Check sheet for the modelled part. Datum: model origin and axes. Units: mm. Face numbers are marked on the shaded views. A direction names the side the tool comes from. Coordinates: 2 decimals unless noted, no trailing zeros. Write each loop counter-clockwise with the first axis right and the second up, starting at its lowest first coordinate (ties: lowest second). Pieces come first, ordered by that corner, then holes. Notation, with made-up numbers: (74, 67) - (96, 67) arc R10 cw to (96, 71) - close; hole circle Ø6 at (-39, 87.25). An arc over 180 degrees is marked (long way). Use one line per item in the form item = value. Start each with the question number.
1. Cross-section at B-B on y = 7. Record the boundary of the cut face in (x, z).
2. Cross-section at C-C on z = -28.8. Record the boundary of the cut face in (x, y).
3. Cross-section at D-D on x = 4.5. Record the boundary of the cut face in (y, z).
4. Tool access check on the marked faces 1, 2 and 3. Record the directions out of +Z, -Z, +X, -X, +Y, -Y that give a thin tool (end or side, any length) a straight path to the whole face; none if there is none.
5. Go/stop test with flat-tipped pins: pin 1 Ø3 at (x, z) = (11, 43) entering from -Y; pin 2 Ø8 at (y, z) = (6, -21.5) entering from -X; pin 3 Ø1.5 at (x, y) = (7.5, 13.5) entering from -Z. Record where each tip stops, or that it passes through.
6. Scan lines: line 1 along Z through (x, y) = (-6.5, 11); line 2 along Z through (x, y) = (15, 6); line 3 along Y through (x, z) = (0.5, 49). Record each from-to range of solid material in increasing order.
7. Cross-section at A-A on x = 0. Record the boundary of the cut face in (y, z), then the cut area to 3 significant figures.
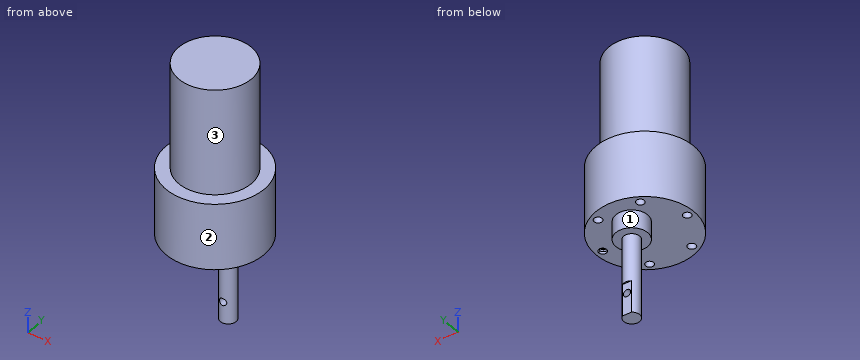
```python
from build123d import *

# Parameters (mm, degrees)
SKETCH1_R           = 18.5
BOSS_EXTRUDE1_DEPTH = 25
SKETCH2_R           = 6
BOSS_EXTRUDE2_DEPTH = 6.8
SKETCH3_R           = 3
BOSS_EXTRUDE3_DEPTH = 30
CUT_EXTRUDE1_DEPTH  = 12
SKETCH5_R           = 13.7
BOSS_EXTRUDE4_DEPTH = 40
SKETCH6_R           = 1.5
CUT_EXTRUDE2_DEPTH  = 3.2
THREAD1_PITCH       = 1.058333333
SKETCH7_R           = 1.350457069
CUT_EXTRUDE3_DEPTH  = 10


with BuildPart() as part:
    # Sketch1 → Boss-Extrude1 (new body)
    with BuildSketch(Plane.XY):
        Circle(SKETCH1_R)
    extrude(amount=BOSS_EXTRUDE1_DEPTH)

    # Sketch2 → Boss-Extrude2 (add)
    with BuildSketch(Plane(origin=(0, 0, 0), x_dir=(-1, 0, 0), z_dir=(0, 0, -1))):
        with Locations(Location((0, 7, 0), (0, 0, 180))):
            Circle(SKETCH2_R)
    extrude(amount=BOSS_EXTRUDE2_DEPTH)

    # Sketch3 → Boss-Extrude3 (add)
    with BuildSketch(Plane(origin=(0, 0, -6.8), x_dir=(-1, 0, 0), z_dir=(0, 0, -1))):
        with Locations((0, 7)):
            Circle(SKETCH3_R)
    extrude(amount=BOSS_EXTRUDE3_DEPTH)

    # Sketch4 → Cut-Extrude1 (cut)
    with BuildSketch(Plane(origin=(0, 0, -36.8), x_dir=(-1, 0, 0), z_dir=(0, 0, -1))):
        Polygon((-80.661429966, 9.5), (-1.658312395, 9.5), (1.658312395, 9.5), (80.661429966, 9.5), (80.661429966, 167.506235142), (-80.661429966, 167.506235142), align=None)
    extrude(amount=-CUT_EXTRUDE1_DEPTH, mode=Mode.SUBTRACT)

    # Sketch5 → Boss-Extrude4 (add)
    with BuildSketch(Plane.XY.offset(25)):
        Circle(SKETCH5_R)
    extrude(amount=BOSS_EXTRUDE4_DEPTH)

    # Sketch6 → Cut-Extrude2 (cut)
    with BuildSketch(Plane(origin=(0, 0, 0), x_dir=(-1, 0, 0), z_dir=(0, 0, -1))):
        with Locations((-15.75, 0)):
            Circle(SKETCH6_R)
        with Locations((-7.875, 13.63990011)):
            Circle(SKETCH6_R)
        with Locations((7.875, 13.63990011)):
            Circle(SKETCH6_R)
        with Locations((15.75, 0)):
            Circle(SKETCH6_R)
        with Locations((7.875, -13.63990011)):
            Circle(SKETCH6_R)
        with Locations((-7.875, -13.63990011)):
            Circle(SKETCH6_R)
    extrude(amount=-CUT_EXTRUDE2_DEPTH, mode=Mode.SUBTRACT)

    # Thread1: the profile of Thread Profile1 profile screwed along a right-hand helix of 3.023622 turns, 8 arcs to a turn; built about Z, then put on its axis
    thread1_z = Axis((0, 0, 0), (0, 0, 1))
    thread1_corners = [(1.5003, 0, -0.000173205), (1.5003, 0, 0.926214869), (0.927160282, 0, 0.595312499), (0.927160282, 0, 0.330729165)]
    with BuildLine(mode=Mode.PRIVATE) as thread1_profile:
        Line(thread1_corners[0], thread1_corners[1])
        Line(thread1_corners[1], thread1_corners[2])
        Line(thread1_corners[2], thread1_corners[3])
        Line(thread1_corners[3], thread1_corners[0])
    thread1_cap = Face(thread1_profile.wire())
    thread1_turn_angles = [0, 22.5, 45, 67.5, 90, 112.5, 135, 157.5, 180, 202.5, 225, 247.5, 270, 292.5, 315, 337.5, 360]
    thread1_turn_weights = [1, 0.9238795325112867, 1, 0.9238795325112867, 1, 0.9238795325112867, 1, 0.9238795325112867, 1, 0.9238795325112867, 1, 0.9238795325112867, 1, 0.9238795325112867, 1, 0.9238795325112867, 1]
    thread1_turn_rails = [Edge.make_bspline([Vector(p[0], p[1], 0).rotate(thread1_z, thread1_turn_angles[k]) / thread1_turn_weights[k] + Vector(0, 0, p[2] + THREAD1_PITCH * thread1_turn_angles[k] / 360) for k in range(17)], [0, 0, 0, 1, 1, 2, 2, 3, 3, 4, 4, 5, 5, 6, 6, 7, 7, 8, 8, 8], 2, thread1_turn_weights) for p in thread1_corners]
    thread1_turn_sides = [Face.make_surface_from_curves(thread1_turn_rails[p[0]], thread1_turn_rails[p[1]]) for p in [(0, 1), (1, 2), (2, 3), (3, 0)]]
    thread1_last_angles = [1080, 1084.251968504, 1088.503937008]
    thread1_last_weights = [1, 0.9972476383747746, 1]
    thread1_last_rails = [Edge.make_bspline([Vector(p[0], p[1], 0).rotate(thread1_z, thread1_last_angles[k]) / thread1_last_weights[k] + Vector(0, 0, p[2] + THREAD1_PITCH * thread1_last_angles[k] / 360) for k in range(3)], [0, 0, 0, 1, 1, 1], 2, thread1_last_weights) for p in thread1_corners]
    thread1_last_sides = [Face.make_surface_from_curves(thread1_last_rails[p[0]], thread1_last_rails[p[1]]) for p in [(0, 1), (1, 2), (2, 3), (3, 0)]]
    thread1 = Plane(origin=(15.75, 0, 0), x_dir=(1, 0, 0), z_dir=(0, 0, 1)) * Solid(Shell([*[p.moved(Location((0, 0, THREAD1_PITCH * i))) for i in range(3) for p in thread1_turn_sides], *thread1_last_sides, thread1_cap, thread1_cap.rotate(thread1_z, 1088.503937008).moved(Location((0, 0, THREAD1_PITCH * 1088.503937008 / 360)))]))
    add(thread1)

    # Sketch7 → Cut-Extrude3 (cut)
    with BuildSketch(Plane(origin=(0, 9.5, 0), x_dir=(1, 0, 0), z_dir=(0, 1, 0))):
        with Locations(Location((0, 28.8, 0), (0, 0, 270))):
            Circle(SKETCH7_R)
    extrude(amount=-CUT_EXTRUDE3_DEPTH, mode=Mode.SUBTRACT)


solid = part.part
```
Final values:
q1.outline = (-17.12, 0) - (-6, 0) - (-6, -6.8) - (-3, -6.8) - (-3, -36.8) - (3, -36.8) - (3, -6.8) - (6, -6.8) - (6, 0) - (17.12, 0) - (17.12, 25) - (11.78, 25) - (11.78, 65) - (-11.78, 65) - (-11.78, 25) - (-17.12, 25) - close; hole circle Ø2.7 at (0, -28.8)
q2.outline = (-1.66, 9.5) arc R3 ccw to (-1.35, 4.32) - (-1.35, 9.5) - close; (1.35, 4.32) arc R3 ccw to (1.66, 9.5) - (1.35, 9.5) - close
q3.outline = (-17.94, 0) - (3.03, 0) - (3.03, -6.8) - (10.97, -6.8) - (10.97, 0) - (17.94, 0) - (17.94, 25) - (12.94, 25) - (12.94, 65) - (-12.94, 65) - (-12.94, 25) - (-17.94, 25) - close
q4.face_1 = -Z
q4.face_2 = +Z, -Z
q4.face_3 = +Z
q5.pin_1 = -9.87
q5.pin_2 = -3
q5.pin_3 = 3.2
q6.line_1 = 0 to 65
q6.line_2 = 0 to 25
q6.line_3 = -13.69 to 13.69
q7.outline = (-18.5, 0) - (1, 0) - (1, -6.8) - (4, -6.8) - (4, -27.45) - (9.5, -27.45) - (9.5, -24.8) - (10, -24.8) - (10, -6.8) - (13, -6.8) - (13, 0) - (18.5, 0) - (18.5, 25) - (13.7, 25) - (13.7, 65) - (-13.7, 65) - (-13.7, 25) - (-18.5, 25) - close; (4, -36.8) - (9.5, -36.8) - (9.5, -30.15) - (4, -30.15) - close
q7.area = 2,260 mm²
